from build123d import *

# Parameters (mm, degrees)
BOSS_EXTRU_1_DEPTH      = 5
ESQUISSE2_W             = 5
ESQUISSE2_H             = 5
ENL_V_MAT_EXTRU_1_DEPTH = 5
ESQUISSE3_W             = 5
ESQUISSE3_H             = 30
BOSS_EXTRU_2_DEPTH      = 5


with BuildPart() as part:
    # Esquisse1 → Boss.-Extru.1 (new body)
    with BuildSketch(Plane.XY):
        with BuildLine():
            Line((-18, 35.436143593), (0, 35.436143593))
            Line((0, 35.436143593), (0, -47.563856407))
            Line((0, -47.563856407), (-18, -47.563856407))
            Line((-18, -47.563856407), (-18, -26.288856407))
            ThreePointArc((-18, -26.288856407), (-3, -11.288856407), (-18, 3.711143593))
            Line((-18, 3.711143593), (-18, 35.436143593))
        make_face()
    extrude(amount=BOSS_EXTRU_1_DEPTH)

    # Esquisse2 → Enlèv. mat.-Extru.1 (cut)
    with BuildSketch(Plane.XY.offset(5)):
        with Locations((-9, 32.936143593)):
            Rectangle(ESQUISSE2_W, ESQUISSE2_H)
        with Locations((-9, -45.063856407)):
            Rectangle(ESQUISSE2_W, ESQUISSE2_H)
    extrude(amount=-ENL_V_MAT_EXTRU_1_DEPTH, mode=Mode.SUBTRACT)

    # Esquisse3 → Boss.-Extru.2 (add)
    with BuildSketch(Plane.XY.offset(5)):
        with Locations((2.5, -11.288856407)):
            Rectangle(ESQUISSE3_W, ESQUISSE3_H)
    extrude(amount=-BOSS_EXTRU_2_DEPTH)


solid = part.part
Geometry check sheet. Reference: the model listing, model coordinates, mm. A direction names the side the tool comes from. Round coordinates to 2 decimals unless told otherwise and drop trailing zeros. Loops run counter-clockwise (first coordinate to the right, second up) from the corner with the lowest first, then second, coordinate; pieces in that order, holes last. Notation, with made-up numbers: (18, 63.25) -> (51, 63.25) arc R30 cw to (51, 98.25) -> close; hole circle Ø7 at (55, 11). An arc over 180 degrees is marked (long way). Answer as a JSON object with one key per item and string values. Group by question number.
Item 1: Cross-section at D-D, the plane x = 1.25. Record the cut outline in (y, z), plus the area to 3 significant figures.
Item 2: Depth check by flat-ended pin: pin 1 Ø2 at (x, z) = (-9.5, 2) entering from -Y; pin 2 Ø3 at (x, y) = (0.5, 14.5) entering from -Z; pin 3 Ø1.5 at (y, z) = (23.5, 2.5) entering from +X; pin 4 Ø1.5 at (x, z) = (-10, 2) entering from +Y. Enter the tip coordinate at first touch or a pass-through.
Item 3: Release check for a two-part mould opening along X. For faces 1 (the face through (-3, 35.436, 2)), 2 (the face through (0, 20, 2)), 3 (the face through (-6.5, -45, 3)), 4 (the face through (-18, -37, 2)) record: pulls with the +X half, pulls with the -X half, needs draft (parallel to the pull), parting line crosses it, or undercut.
Item 4: Cross-section at C-C, the plane x = -7.75. Record the cut outline in (y, z).
Item 5: Cross-section at B-B, the plane z = 1.15. Record the cut outline in (x, y).
Item 6: Cross-section at A-A, the plane x = -16.5. Record the cut outline in (y, z).
Item 7: Set-up check for faces 5 (the face through (2, 3.711, 3)), 6 (the face through (-6.5, 33, 3)), 7 (the face through (-11.5, -45, 3)), 8 (the face through (0, -37, 2)): record each of +Z, -Z, +X, -X, +Y, -Y from which the full face is reachable in a straight line by a thin tool's end or side.
Item 8: Thickness scan on line 1 along X through (y, z) = (-34, 4.4); line 2 along Y through (x, z) = (1, 4.45); line 3 along Y through (x, z) = (-10.5, 4.2). Record the ranges inside material, lowest first.
Determined:
{
 "1": {"outline": "(-26.29, 0) -> (3.71, 0) -> (3.71, 5) -> (-26.29, 5) -> close", "area": "150 mm²"},
 "2": {"pin 1": "stops at y = -42.56", "pin 2": "stops at z = 0", "pin 3": "stops at x = 0", "pin 4": "stops at y = 30.44"},
 "3": {"face 1": "needs draft", "face 2": "pulls with the +X half", "face 3": "undercut", "face 4": "pulls with the -X half"},
 "4": {"outline": "(-42.56, 0) -> (-22.24, 0) -> (-22.24, 5) -> (-42.56, 5) -> close; (-0.34, 0) -> (30.44, 0) -> (30.44, 5) -> (-0.34, 5) -> close"},
 "5": {"outline": "(-18, -47.56) -> (-11.5, -47.56) -> (-11.5, -42.56) -> (-6.5, -42.56) -> (-6.5, -47.56) -> (0, -47.56) -> (0, -26.29) -> (5, -26.29) -> (5, 3.71) -> (0, 3.71) -> (0, 35.44) -> (-6.5, 35.44) -> (-6.5, 30.44) -> (-11.5, 30.44) -> (-11.5, 35.44) -> (-18, 35.44) -> (-18, 3.71) arc R15 cw to (-18, -26.29) -> close"},
 "6": {"outline": "(-47.56, 0) -> (-26.21, 0) -> (-26.21, 5) -> (-47.56, 5) -> close; (3.64, 0) -> (35.44, 0) -> (35.44, 5) -> (3.64, 5) -> close"},
 "7": {"face 5": "+Z, -Z, +X, +Y", "face 6": "+Z, -Z, +Y", "face 7": "+Z, -Z, -Y", "face 8": "+Z, -Z, +X, -Y"},
 "8": {"line 1": "x = -18 to 0", "line 2": "y = -26.29 to 3.71", "line 3": "y = -42.56 to -24.28, 1.7 to 30.44"}
}
